Verification items for the finished model (mm, model axes). Face numbers are marked on the shaded views. A direction names the side the tool comes from. Coordinates: 2 decimals unless noted, no trailing zeros. Order: outer loops, then holes, each group sorted by start corner. A loop starts at its lowest first (then second) coordinate and runs counter-clockwise, first axis right, second up. Notation, with made-up numbers: M 30,25 L 45,25 A33 ccw 45,64 Z; hole C -13.5,3 d8. An arc over 180 degrees is marked long. Return JSON: item names as keys, results as strings.
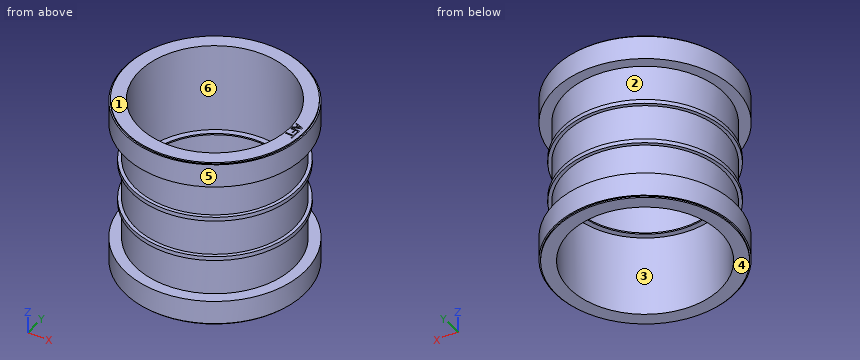
Autodesk Inventor part; units mm, degrees
ref_plane "YZ Plane" through (0, 0, 0) normal (1, 0, 0) x (0, 1, 0)
ref_plane "XZ Plane" through (0, 0, 0) normal (0, 1, 0) x (-1, 0, 0)
ref_plane "XY Plane" through (0, 0, 0) normal (0, 0, 1) x (1, 0, 0)
sketch "Sketch1" plane through (0, 0, 0) normal (1, 0, 0) x (0, 1, 0)
  line L0 (0, 0) -> (0, -141.6259) construction
  line L1 (-13.3, 0) -> (79.8, 0) construction
  line L2 (55.5, -66.5) -> (25.7904, -66.5) construction
  line L3 (51.5, -66) -> (51.5, -67)
  line L4 (51.5, -66) -> (55.5, -66)
  line L5 (55.5, -66) -> (55.5, 0)
  line L6 (51.5, -67) -> (55.5, -67)
  line L7 (55.5, -67) -> (55.5, -127)
  line L8 (66.5, -108.5) -> (58.5, -108.5)
  line L9 (58.5, -108.5) -> (58.5, -80.5)
  line L10 (58.5, -80.5) -> (61, -80.5)
  line L11 (61, -80.5) -> (61, -77.5)
  line L12 (61, -77.5) -> (58.5, -77.5)
  line L13 (58.5, -77.5) -> (58.5, -49.5)
  line L14 (58.5, -49.5) -> (61, -49.5)
  line L15 (61, -49.5) -> (61, -46.5)
  line L16 (61, -46.5) -> (58.5, -46.5)
  line L17 (58.5, -46.5) -> (58.5, -18.5)
  line L18 (58.5, -18.5) -> (66.5, -18.5)
  line L19 (66.5, -18.5) -> (66.5, -1)
  line L20 (66.5, -1) -> (65.5, -1)
  line L21 (65.5, -1) -> (65.5, 0)
  line L22 (65.5, 0) -> (55.5, 0)
  line L23 (66.5, -108.5) -> (66.5, -126)
  line L24 (66.5, -126) -> (65.5, -126)
  line L25 (65.5, -126) -> (65.5, -127)
  line L26 (65.5, -127) -> (55.5, -127)
  point P0 (51.5, -66.5)
  dimension "d2" = 1
  dimension "d3" = 103
  dimension "d4" = 66
  dimension "d5" = 111
  dimension "d6" = 60
  dimension "d9" = 8
  dimension "d10" = 28
  dimension "d11" = 2.5
  dimension "d12" = 3
  dimension "d13" = 28
  dimension "d14" = 2.5
  dimension "d15" = 3
  dimension "d16" = 28
  dimension "d17" = 8
  dimension "d19" = 17.5
  dimension "d20" = 1
  dimension "d21" = 17.5
  dimension "d22" = 1
  dimension "d23" = 3
  dimension "d24" = 1
  dimension "d25" = 1
revolve "Revolution1" add sketch "Sketch1" angle 360 about axis through (0, 0, 0) along (0, 0, -1)
sketch "Sketch2" plane through (0, 0, 0) normal (0, 0, 1) x (1, 0, 0)
  line L0 (62.3533, 7.1392) -> (62.3533, -1.0719) construction
  line L1 (62.3533, -1.0719) -> (58.8533, -1.0719) construction
  line L2 (58.8533, -1.0719) -> (58.8533, 7.1392) construction
  line L3 (58.8533, 7.1392) -> (62.3533, 7.1392) construction
  line L4 (56.2533, 7.1788) -> (62.3533, 5.1223)
  line L5 (62.3533, 5.1223) -> (62.3533, 4.1238)
  line L6 (62.3533, 4.1238) -> (56.2533, 2.0674)
  line L7 (56.2533, 2.0674) -> (56.2533, 2.9226)
  line L8 (56.2533, 2.9226) -> (57.9587, 3.4762)
  line L9 (57.9587, 3.4762) -> (57.9587, 5.8045)
  line L10 (57.9587, 5.8045) -> (56.2533, 6.3582)
  line L11 (56.2533, 6.3582) -> (56.2533, 7.1788)
  line L12 (58.6507, 3.6987) -> (61.5228, 4.6429)
  line L13 (61.5228, 4.6429) -> (58.6507, 5.5821)
  line L14 (58.6507, 5.5821) -> (58.6507, 3.6987)
  line L15 (61.6315, -2.1591) -> (61.6315, 0.6783)
  line L16 (61.6315, 0.6783) -> (59.9113, 0.6783)
  line L17 (59.9113, 0.6783) -> (59.9113, -2.0405)
  line L18 (59.9113, -2.0405) -> (59.1896, -2.0405)
  line L19 (59.1896, -2.0405) -> (59.1896, 0.6783)
  line L20 (59.1896, 0.6783) -> (56.2533, 0.6783)
  line L21 (56.2533, 0.6783) -> (56.2533, 1.489)
  line L22 (56.2533, 1.489) -> (62.3533, 1.489)
  line L23 (62.3533, 1.489) -> (62.3533, -2.1591)
  line L24 (62.3533, -2.1591) -> (61.6315, -2.1591)
  line L25 (56.2533, -4.3094) -> (61.6315, -4.3094)
  line L26 (61.6315, -4.3094) -> (61.6315, -2.2629)
  line L27 (61.6315, -2.2629) -> (62.3533, -2.2629)
  line L28 (62.3533, -2.2629) -> (62.3533, -7.1666)
  line L29 (62.3533, -7.1666) -> (61.6315, -7.1666)
  line L30 (61.6315, -7.1666) -> (61.6315, -5.1201)
  line L31 (61.6315, -5.1201) -> (56.2533, -5.1201)
  line L32 (56.2533, -5.1201) -> (56.2533, -4.3094)
  point P0 (0, 0)
emboss "Emboss1" sketch "Sketch2" operation cut depth 0.001 direction (0, 0, -1)
equation "\"d22\" = d20"
equation "\"d24\" = d20"
equation "\"d25\" = d24"
properties part number "doubleSocketPipe" material "PVC-Piping"
Q1. Draft check along X on the marked faces 4, 5 and 6. Enter one of: pulls with the +X half, pulls with the -X half, needs draft (parallel to the pull), parting line crosses it, or undercut.
Values:
{"face 4": "needs draft", "face 5": "parting line crosses it", "face 6": "undercut"}
Q2. Go/stop test with flat-tipped pins: pin 1 (6 mm diameter, centred on x = 21, z = -27, fed in from -Y); pin 2 (5 mm diameter, centred on x = -14, z = -34.5, fed in from -Y); pin 3 (1 mm diameter, centred on y = 50.5, z = -102, fed in from -X). Record where each tip stops, or that it passes through.
Values:
{"pin 1": "y = -55.66", "pin 2": "y = -57.36", "pin 3": "x = -30.37"}
Q3. Tool access check on the marked faces 1, 2 and 3. Record the directions out of +Z, -Z, +X, -X, +Y, -Y that give a thin tool (end or side, any length) a straight path to the whole face; none if there is none.
Values:
{"face 1": "+Z, +X, -X, +Y, -Y", "face 2": "none", "face 3": "-Z"}
Q4. Cross-section at A-A, the plane z = -73. Record the boundary of the cut face in (x, y), and give its area (3 significant figures).
Values:
{"outline": "C 0,0 d117; hole C 0,0 d111", "area": "1,070 mm^2"}
Q5. Cross-section at B-B, the plane z = -110.5. Record the boundary of the cut face in (x, y).
Values:
{"outline": "C 0,0 d133; hole C 0,0 d111"}
Q6. Material ranges on line 1 along Z through (x, y) = (-3.5, -60.5); line 2 along Y through (x, z) = (1, -104); line 3 along Z through (x, y) = (43, -49), recorded low to high.
Values:
{"line 1": "-127 to -108.5, -80.5 to -77.5, -49.5 to -46.5, -18.5 to 0", "line 2": "-58.49 to -55.49, 55.49 to 58.49", "line 3": "-127 to -108.5, -18.5 to 0"}
